For this review, take the finished solid that the model builds, in its own axes (mm). A direction names the side the tool comes from. Coordinates: 2 decimals unless noted, no trailing zeros. Order: outer loops, then holes, each group sorted by start corner. A loop starts at its lowest first (then second) coordinate and runs counter-clockwise, first axis right, second up. Notation, with made-up numbers: M -8.5,46.25 L 39.5,46.25 A25 cw 39.5,71.25 Z; hole C 36,7.25 d4. An arc over 180 degrees is marked long. Use CSV: the item, a comma, the result in double quotes.
Autodesk Inventor part; units mm, degrees
ref_plane "Work Plane1" through (-1.27, 0, 3.94) normal (0, 0, 1) x (1, 0, 0)
ref_plane "YZ Plane" through (0, 0, 0) normal (1, 0, 0) x (0, 1, 0)
ref_plane "XZ Plane" through (0, 0, 0) normal (0, 1, 0) x (-1, 0, 0)
sketch "Sketch1" plane through (0, 0, 0) normal (0, 1, 0) x (-1, 0, 0)
  line L0 (-1.27, -4.065) -> (-1.27, 4.065)
  line L1 (-1.27, 4.065) -> (1.27, 4.065)
  line L2 (1.27, 4.065) -> (1.27, -4.065)
  line L3 (1.0272, -4.065) -> (0.8972, -3.935)
  line L4 (0.8972, -3.935) -> (-0.8972, -3.935)
  line L5 (-0.8972, -3.935) -> (-1.0272, -4.065)
  line L6 (1.27, -4.065) -> (1.0272, -4.065)
  line L7 (-1.0272, -4.065) -> (-1.27, -4.065)
  line L8 (0, -2.6831) -> (0, -0.9898) construction
  point P0 (0, 0)
  point P1 (0, 4.065)
  point P2 (1.27, 0)
  point P3 (0, -3.935)
  dimension "d1" = 2.54
  dimension "d2" = 0.13
  dimension "d3" = 8.13
  dimension "d4" = 45
extrude "Extrusion1" add sketch "Sketch1" along normal blind 5.08
sketch "Sketch2" plane through (-1.27, 0, 4.065) normal (0, 0, 1) x (1, 0, 0)
  line L0 (0.825, 4.255) -> (1.715, 4.255)
  line L1 (1.715, 4.255) -> (1.715, 3.365)
  line L2 (1.715, 3.365) -> (0.825, 3.365)
  line L3 (0.825, 3.365) -> (0.825, 4.255)
  line L4 (0.825, 1.715) -> (1.715, 1.715)
  line L5 (1.715, 1.715) -> (1.715, 0.825)
  line L6 (1.715, 0.825) -> (0.825, 0.825)
  line L7 (0.825, 0.825) -> (0.825, 1.715)
  line L8 (0.4511, 3.81) -> (2.2201, 3.81) construction
  line L9 (2.2201, 1.27) -> (0.4335, 1.27) construction
  line L10 (0, 0) -> (2.54, 0)
  line L11 (2.54, 0) -> (2.54, 5.08)
  line L12 (0, 5.08) -> (2.54, 5.08)
  line L13 (0, 0) -> (0, 5.08)
  point P0 (1.27, 0)
  point P1 (0.825, 3.81)
  point P2 (0.825, 1.27)
  point P3 (1.27, 5.08)
  point P4 (1.27, 4.255)
  point P5 (1.27, 1.715)
  dimension "d7" = 2.54
  dimension "d8" = 0.89
  dimension "d9" = 1.27
extrude "Extrusion2" cut sketch "Sketch2" against normal blind 8 contours L0 L1 L2 L3 | L4 L5 L6 L7
sketch "Sketch3" plane through (0, 0, 0) normal (1, 0, 0) x (0, 1, 0)
  line L0 (0, 4.065) -> (5.08, 4.065)
  line L1 (5.08, -4.065) -> (5.08, 4.065)
  line L2 (0, -3.935) -> (5.08, -3.935)
  line L3 (-0.39, 5.59) -> (-0.64, 5.59)
  line L4 (-0.64, 5.59) -> (-0.64, 3.7923)
  line L5 (-0.64, 3.7923) -> (-0.2868, 3.7923)
  line L6 (-0.39, 4.0423) -> (-0.39, 5.59)
  line L7 (-0.39, -3.7923) -> (-0.64, -3.7923)
  line L8 (-0.64, -3.7923) -> (-0.64, -5.59)
  line L9 (-0.64, -5.59) -> (-0.39, -5.59)
  line L10 (-0.39, -5.59) -> (-0.39, -4.0423)
  line L11 (-1.3876, 0) -> (-0.3881, 0) construction
  line L12 (0, -4.065) -> (0, 4.065)
  line L13 (-0.39, -3.7923) -> (0, -3.7923)
  line L14 (0, -3.7923) -> (0, -4.0423)
  line L15 (0, -4.0423) -> (-0.39, -4.0423)
  line L16 (-0.39, 4.0423) -> (0, 4.0423)
  line L17 (0, 4.0423) -> (0, 3.7923)
  line L18 (0, 3.7923) -> (-0.2868, 3.7923)
  point P0 (0, 0)
  dimension "d30" = 0.25
  dimension "d31" = 11.18
  dimension "d34" = 5.72
ref_plane "Work Plane1" through (-1.27, 0, 3.94) normal (0, 0, 1) x (1, 0, 0)
extrude "Extrusion3" add sketch "Sketch3" along normal mid plane 0.51 contours L12 L18 L5 L4 L3 L6 L16 | L12 L15 L10 L9 L8 L7 L13
chamfer "Chamfer1" distance 0.5 angle 45 8 edges at (0.445, 3.81, 4.065) (0, 3.365, 4.065) (-0.445, 3.81, 4.065) (0, 4.255, 4.065) (0, 1.715, 4.065) (0.445, 1.27, 4.065) (0, 0.825, 4.065) (-0.445, 1.27, 4.065)
ref_plane "Work Plane3" through (-0.255, -0.64, 0) normal (0, 0, 1) x (1, 0, 0)
sketch "Sketch6" plane through (0, 0, 0) normal (0, -1, 0) x (1, 0, 0)
  line L0 (0.255, -3.7923) -> (0.255, -3.935)
  line L1 (0.8972, -3.935) -> (0.255, -3.935)
  line L2 (1.0272, -4.065) -> (0.8972, -3.935)
  line L3 (1.27, -4.065) -> (1.0272, -4.065)
  line L4 (1.27, 4.065) -> (1.27, -4.065)
  line L5 (-1.27, 4.065) -> (1.27, 4.065)
  line L6 (-1.27, -4.065) -> (-1.27, 4.065)
  line L7 (-1.0272, -4.065) -> (-1.27, -4.065)
  line L8 (-0.8972, -3.935) -> (-1.0272, -4.065)
  line L9 (-0.255, -3.935) -> (-0.8972, -3.935)
  line L10 (-0.255, -3.935) -> (-0.255, -3.7923)
  line L11 (-0.255, -3.7923) -> (0.255, -3.7923)
  line L12 (-0.255, 3.7923) -> (-0.255, 4.0423)
  line L13 (-0.255, 4.0423) -> (0.255, 4.0423)
  line L14 (0.255, 4.0423) -> (0.255, 3.7923)
  line L15 (0.255, 3.7923) -> (-0.255, 3.7923)
  point P0 (0, 0)
extrude "Extrusion4" add sketch "Sketch6" along normal blind 0.65
properties part number "SSM-101-F-DH"
Item 1: Add section C-C on z = 2.5. State the section outline as (x, y) points (3 decimals).
Solutions:
outline,"M -1.27,-0.65 L 1.27,-0.65 L 1.27,5.08 L -1.27,5.08 Z; hole M -0.445,0.825 L 0.445,0.825 L 0.445,1.715 L -0.445,1.715 Z; hole M -0.445,3.365 L 0.445,3.365 L 0.445,4.255 L -0.445,4.255 Z"
Item 2: Draft analysis for pull direction X (two halves, no side actions). For faces 3 (the face through (0, -0.65, 0)), 4 (the face through (1.27, 2, 0)), 5 (the face through (-0.445, 4, 0)), state which applies: released by +X, released by -X, zero draft, split by the parting line, or undercut.
Solutions:
face 3,"zero draft"
face 4,"released by +X"
face 5,"undercut"
Item 3: For faces 1 (the face through (0, 5.08, 0)), 2 (the face through (0, 0.825, 0)), list the 3-axis set-ups (+Z, -Z, +X, -X, +Y, -Y) from which the entire face can be reached by the end or side of a thin tool; tool diameter is ignored.
Solutions:
face 1,"+Z, -Z, +X, -X, +Y"
face 2,"+Z, -Z"
Item 4: Add section D-D on y = -0.25. State the section outline as (x, z) points (3 decimals).
Solutions:
outline,"M -1.27,-4.065 L -1.027,-4.065 L -0.897,-3.935 L -0.255,-3.935 L -0.255,-4.042 L 0.255,-4.042 L 0.255,-3.935 L 0.897,-3.935 L 1.027,-4.065 L 1.27,-4.065 L 1.27,4.065 L -1.27,4.065 Z"
Item 5: To check wall thickness, follow line 1 along X through (y, z) = (4, 3) (3 decimals); line 2 along Y through (x, z) = (-0.05, -0.5) (3 decimals); line 3 along Z through (x, y) = (0.5, 4.8) (3 decimals). State the ranges of each line that lie inside material, in increasing order. Write a range as [from, to].
Solutions:
line 1,"[-1.27, -0.445], [0.445, 1.27]"
line 2,"[-0.65, 0.825], [1.715, 3.365], [4.255, 5.08]"
line 3,"[-3.935, 4.065]"
Item 6: Add section A-A on y = 3.6. State the section outline as (x, z) points (3 decimals).
Solutions:
outline,"M -1.27,-4.065 L -1.027,-4.065 L -0.897,-3.935 L -0.445,-3.935 L -0.445,3.565 L -0.945,4.065 L -1.27,4.065 Z; M 0.445,-3.935 L 0.897,-3.935 L 1.027,-4.065 L 1.27,-4.065 L 1.27,4.065 L 0.945,4.065 L 0.445,3.565 Z"
Item 7: Add section B-B on x = 0.15. State how many separate pieces and enclosed holes the cut face has, and give its area (3 significant figures).
Solutions:
separate pieces,"3"
enclosed holes,"0"
area,"31.9 mm^2"
Item 8: Clearance check with flat-ended pins moving along their axes: pin 1 Ø0.5 at (y, z) = (0, -4.5) entering from -X; pin 2 Ø1 at (x, y) = (0, 2.5) entering from +Z (3 decimals). State where each tip first meets the part, or that it passes through.
Solutions:
pin 1,"through"
pin 2,"z = 4.065"
